Can you work these out from the model? Positions are in its coordinate system, mm. Round coordinates to 2 decimals unless told otherwise and drop trailing zeros. Write each loop counter-clockwise with the first axis right and the second up, starting at its lowest first coordinate (ties: lowest second). Pieces come first, ordered by that corner, then holes.
Q1. If we section it at B-B (x = 135): Please give me the cut outline in (y, z), plus the area to 3 significant figures.
Q2. I'm going to push a flat-ended pin straight in: pin 1 Ø1.5 at (x, z) = (108, 1) entering from -Y. Where does the tip first touch, or does it pass through?
Q3. If we section it at C-C (y = 271.5): Please give me the cut outline in (x, z), plus the area to 3 significant figures.
Q4. If we section it at A-A (z = 1.85): Please give me the cut outline in (x, y), plus the area to 3 significant figures.
Q5. Please list where these lines run through material, in increasing order: line 1 along Y through (x, z) = (75, 2.15); line 2 along X through (y, z) = (145, 1.1); line 3 along Y through (x, z) = (126, 0.3).
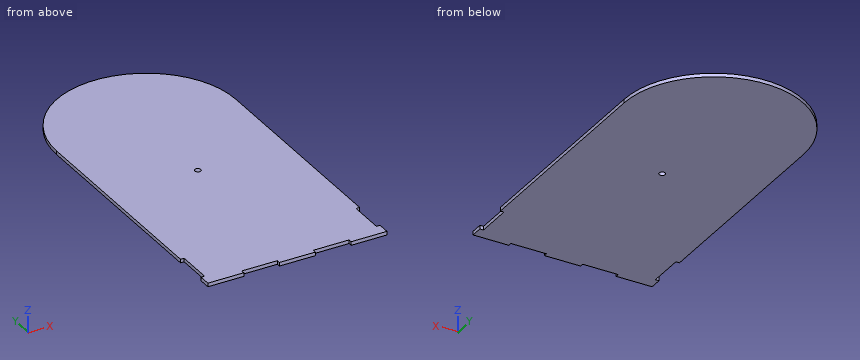
from build123d import *

# Parameters (mm, degrees)
SKETCH1_R           = 2.5
BOSS_EXTRUDE1_DEPTH = 3


with BuildPart() as part:
    # Sketch1 → Boss-Extrude1 (new body)
    with BuildSketch(Plane.XY):
        with BuildLine():
            Line((59.9, 0), (90.1, 0))
            Line((90.1, 0), (90.1, 3))
            Line((90.1, 3), (119.9, 3))
            Line((119.9, 3), (119.9, 0))
            Line((119.9, 0), (150, 0))
            Line((150, 0), (150, 10))
            Line((150, 10), (147, 10))
            Line((147, 10), (147, 39.8))
            Line((147, 39.8), (150, 39.8))
            Line((150, 39.8), (150, 220))
            ThreePointArc((150, 220), (75, 295), (0, 220))
            Line((0, 220), (0, 39.8))
            Line((0, 39.8), (3, 39.8))
            Line((3, 39.8), (3, 10))
            Line((3, 10), (0, 10))
            Line((0, 10), (0, 0))
            Line((0, 0), (30.1, 0))
            Line((30.1, 0), (30.1, 3))
            Line((30.1, 3), (59.9, 3))
            Line((59.9, 3), (59.9, 0))
        make_face()
        with Locations((75, 145)):
            Circle(SKETCH1_R, mode=Mode.SUBTRACT)
    extrude(amount=BOSS_EXTRUDE1_DEPTH)


solid = part.part
A:
1. outline: (0, 0) - (265, 0) - (265, 3) - (0, 3) - close
1. area: 795 mm2
2. pin 1: stops at y = 3
3. outline: (20.48, 0) - (129.52, 0) - (129.52, 3) - (20.48, 3) - close
3. area: 327 mm2
4. outline: (0, 0) - (30.1, 0) - (30.1, 3) - (59.9, 3) - (59.9, 0) - (90.1, 0) - (90.1, 3) - (119.9, 3) - (119.9, 0) - (150, 0) - (150, 10) - (147, 10) - (147, 39.8) - (150, 39.8) - (150, 220) arc R75 ccw to (0, 220) - (0, 39.8) - (3, 39.8) - (3, 10) - (0, 10) - close; hole circle Ø5 at (75, 145)
4. area: 41,500 mm2
5. line 1: y = 0 to 142.5, 147.5 to 295
5. line 2: x = 0 to 72.5, 77.5 to 150
5. line 3: y = 0 to 274.99
